Part model, mm, in its own coordinate system. A direction names the side the tool comes from. Give positions to 0.01 mm unless a question says otherwise; leave off trailing zeros. Order: outer loops, then holes, each group sorted by start corner. A loop starts at its lowest first (then second) coordinate and runs counter-clockwise, first axis right, second up. Notation, with made-up numbers: (18.25, 28) - (69.25, 28) arc R13 ccw to (69.25, 53) - close; hole circle Ø5 at (66, 42.25). An arc over 180 degrees is marked (long way). One line per item, written item: value.
```python
from build123d import *

# Parameters (mm, degrees)
BOSS_EXTRUDE1_DEPTH = 3.175
SKETCH2_R           = 1.6
CUT_EXTRUDE1_DEPTH  = 25.914265492
CUT_EXTRUDE2_DEPTH  = 25.914265492


with BuildPart() as part:
    # Sketch1 → Boss-Extrude1 (new body)
    with BuildSketch(Plane(origin=(0, 0, 0), x_dir=(1, 0, 0), z_dir=(0, 1, 0))):
        with BuildLine():
            Line((-4.196638655, 20.168), (-4.995998399, 0.2))
            ThreePointArc((-4.995998399, 0.2), (0, -5), (4.995998399, 0.2))
            Line((4.995998399, 0.2), (4.196638655, 20.168))
            ThreePointArc((4.196638655, 20.168), (0, 24.2), (-4.196638655, 20.168))
        make_face()
    extrude(amount=BOSS_EXTRUDE1_DEPTH)

    # Sketch2 → Cut-Extrude1 (cut, through all)
    with BuildSketch(Plane(origin=(0, 3.175, 0), x_dir=(1, 0, 0), z_dir=(0, 1, 0))):
        with Locations(Location((0, 0, 0), (0, 0, 270))):
            Circle(SKETCH2_R)
        with Locations(Location((0, 10, 0), (0, 0, 270))):
            Circle(SKETCH2_R)
    extrude(amount=-CUT_EXTRUDE1_DEPTH, mode=Mode.SUBTRACT)

    # Sketch3 → Cut-Extrude2 (cut, through all)
    with BuildSketch(Plane(origin=(0, 3.175, 0), x_dir=(1, 0, 0), z_dir=(0, 1, 0))):
        with BuildLine():
            Line((-2.2, 16.5), (-2.2, 20))
            ThreePointArc((-2.2, 20), (0, 22.2), (2.2, 20))
            Line((2.2, 20), (2.2, 16.5))
            ThreePointArc((2.2, 16.5), (0, 14.3), (-2.2, 16.5))
        make_face()
    extrude(amount=-CUT_EXTRUDE2_DEPTH, mode=Mode.SUBTRACT)


solid = part.part
```
1) Mould opens along X. For faces 3 (the cylindrical face through (0, 1.6, -14.3)), 4 (the cylindrical face through (0.1, 1.6, -24.2)), 5 (the flat face through (0, 3.175, -7)) say: released by +X, released by -X, zero draft, split by the parting line, or undercut.
Outcome:
face 3: undercut
face 4: split by the parting line
face 5: zero draft
2) Cut at C-C, the plane z = -10. Give the cut face in (x, y) (3 decimals), then the cut area to 3 significant figures.
Outcome:
outline: (-4.604, 0) - (-1.6, 0) - (-1.6, 3.175) - (-4.604, 3.175) - close; (1.6, 0) - (4.604, 0) - (4.604, 3.175) - (1.6, 3.175) - close
area: 19.1 mm^2
3) Which spindle directions (+Z, -Z, +X, -X, +Y, -Y) get a long thin tool onto all of the face, cutting with end or side? Do faces 1 (the flat face through (-4.59, 1.57, -10.32)), 2 (the flat face through (-2.2, 2, -18)). Say none if no direction does.
Outcome:
face 1: -Z, -X, +Y, -Y
face 2: +Y, -Y
4) Cut at D-D, the plane x = -1.25. Give the cut face in (y, z) (3 decimals).
Outcome:
outline: (0, -24.01) - (3.175, -24.01) - (3.175, -21.81) - (0, -21.81) - close; (0, -14.69) - (3.175, -14.69) - (3.175, -10.999) - (0, -10.999) - close; (0, -9.001) - (3.175, -9.001) - (3.175, -0.999) - (0, -0.999) - close; (0, 0.999) - (3.175, 0.999) - (3.175, 4.841) - (0, 4.841) - close
5) Cut at A-A, the plane x = 0. Give the cut face in (y, z) (3 decimals).
Outcome:
outline: (0, -24.2) - (3.175, -24.2) - (3.175, -22.2) - (0, -22.2) - close; (0, -14.3) - (3.175, -14.3) - (3.175, -11.6) - (0, -11.6) - close; (0, -8.4) - (3.175, -8.4) - (3.175, -1.6) - (0, -1.6) - close; (0, 1.6) - (3.175, 1.6) - (3.175, 5) - (0, 5) - close
6) Cut at B-B, the plane y = 0.4. Give the cut face in (x, z).
Outcome:
outline: (-5, -0.2) - (-4.2, -20.17) arc R4.2 ccw to (4.2, -20.17) - (5, -0.2) arc R5 ccw (long way) to start; hole (-2.2, -20) arc R2.2 ccw to (2.2, -20) - (2.2, -16.5) arc R2.2 ccw to (-2.2, -16.5) - close; hole circle Ø3.2 at (0, -10); hole circle Ø3.2 at (0, 0)
7) Drill centre lines: line 1 along X through (y, z) = (1.55, 0); line 2 along X through (y, z) = (1.9, -15.75); line 3 along Z through (x, y) = (-2.75, 1.9). Where is each one in solid material? Low to high. Write a range as from..to.
Outcome:
line 1: x = -5..-1.6, 1.6..5
line 2: x = -4.37..-2.07, 2.07..4.37
line 3: z = -23.17..4.18
8) Pin check, flat tip, straight feed: pin 1 (1.5 mm diameter, centred on y = 0.5, z = -7, fed in from -X). Stop position of the tip, or through.
Outcome:
pin 1: stops at x = -4.75
